Can you work these out from the model? Positions are in its coordinate system, mm. A direction names the side the tool comes from. Give positions to 0.01 mm unless a question says otherwise; leave off trailing zeros. Loops run counter-clockwise (first coordinate to the right, second up) from the corner with the lowest first, then second, coordinate; pieces in that order, holes last. Notation, with made-up numbers: (-0.75, 14.5) - (12.25, 14.5) arc R28 ccw to (12.25, 47.5) - close; hole circle Ø11 at (-21.5, 18.5). An arc over 180 degrees is marked (long way). Answer as a JSON object with one key per item and string values. Group by question number.
Item 1: Suppose I cut it at C-C on z = 7. Write out the boundary of the cut face in (x, y), and give its area (3 significant figures).
Item 2: Will these pins go through, and if not, where does the flat tip stop? pin 1 (12.5 mm diameter, centred on x = -25.5, z = -1.5, fed in from -Y); pin 2 (1.6 mm diameter, centred on x = 1, z = -3, fed in from +Y); pin 3 (1.7 mm diameter, centred on y = 3.5, z = -4.5, fed in from -X).
Item 3: Which directions (+Z, -Z, +X, -X, +Y, -Y) give clear straight access to the entire face, cutting with the end or side of a thin tool? Please do faces 4 (the flat face through (25, 3, -1.687)), 5 (the flat face through (-0.3, 2.8, -15.3)), 6 (the flat face through (-24, 4, -12.057)).
Item 4: Suppose I cut it at A-A on x = -22. Write out the boundary of the cut face in (y, z), and give its area (3 significant figures).
Item 5: Thinking about a two-plate mould opening in X: for faces 1 (the flat face through (-24, 13.04, -3)), 2 (the flat face through (-31.554, 4.42, -10.79)), 3 (the flat face through (-3, 1.6, -3)), which applies, pulls with the +X half, pulls with the -X half, needs draft (parallel to the pull), parting line crosses it, or undercut?
Item 6: Please list where these lines run through material, in increasing order: L1, parallel to X at y = 3, z = 2; L2, parallel to Y at x = -28.5, z = -2; L3, parallel to X at y = 3.5, z = -14.
Item 7: Suppose I cut it at B-B on x = 14. Write out the boundary of the cut face in (y, z).
Item 8: Suppose I cut it at D-D on y = 10. Write out the boundary of the cut face in (x, z), and give its area (3 significant figures).
from build123d import *

# Parameters (mm, degrees)
SKETCH_1_W          = 65
SKETCH_1_H          = 30.64
EXTRUDE_1_DEPTH     = 1.6
FILLET_1_R          = 2
SKETCH_2_R          = 1.35
CUT_EXTRUDE_1_DEPTH = 1.6
SKETCH_3_W          = 51.3
SKETCH_3_H          = 5
EXTRUDE_2_DEPTH     = 4
SKETCH_4_W          = 17.3
SKETCH_4_H          = 17.3
EXTRUDE_3_DEPTH     = 5.72
CHAMFER_1_SIZE      = 2.5
SKETCH_5_R          = 6.95
EXTRUDE_4_DEPTH     = 1
SKETCH_6_R          = 1.326147724
EXTRUDE_5_DEPTH     = 3.72
SKETCH_7_R          = 5.6
EXTRUDE_6_DEPTH     = 1
SKETCH_8_W          = 6.2
SKETCH_8_H          = 6.2
EXTRUDE_7_DEPTH     = 2
SKETCH_9_R          = 1.56
EXTRUDE_8_DEPTH     = 1
SKETCH_10_W         = 3.44
SKETCH_10_H         = 3
EXTRUDE_9_DEPTH     = 1.2
SKETCH_11_R         = 0.875
EXTRUDE_10_DEPTH    = 0.5


with BuildPart() as part:
    # 草图1 → 凸台-拉伸1 (new body)
    with BuildSketch(Plane(origin=(0, 0, 0), x_dir=(1, 0, 0), z_dir=(0, 1, 0))):
        with Locations((-2.796247961, 2.767463295)):
            Rectangle(SKETCH_1_W, SKETCH_1_H)
    extrude(amount=EXTRUDE_1_DEPTH)

    # 圆角1
    fillet_1_edges = [part.edges().sort_by_distance(p)[0] for p in [
        (-35.296247961, 0.8, -18.087463295),
        (29.703752039, 0.8, -18.087463295),
        (29.703752039, 0.8, 12.552536705),
        (-35.296247961, 0.8, 12.552536705),
    ]]
    fillet(fillet_1_edges, radius=FILLET_1_R)

    # 草图2 → 切除-拉伸1 (cut)
    with BuildSketch(Plane(origin=(0, 1.6, 0), x_dir=(1, 0, 0), z_dir=(0, 1, 0))):
        with Locations(Location((-32.996247961, 15.787463295, 0), (0, 0, 270))):  # turned: the seam where the file's is
            Circle(SKETCH_2_R)
        with Locations(Location((27.403752039, 15.787463295, 0), (0, 0, 270))):  # turned: the seam where the file's is
            Circle(SKETCH_2_R)
        with Locations(Location((27.403752039, -9.702536705, 0), (0, 0, 270))):  # turned: the seam where the file's is
            Circle(SKETCH_2_R)
        with Locations(Location((-32.996247961, -9.702536705, 0), (0, 0, 270))):  # turned: the seam where the file's is
            Circle(SKETCH_2_R)
    extrude(amount=-CUT_EXTRUDE_1_DEPTH, mode=Mode.SUBTRACT)

    # 草图3 → 凸台-拉伸2 (add)
    with BuildSketch(Plane.XZ):
        with Locations((-2.446247961, 8.452536705)):
            Rectangle(SKETCH_3_W, SKETCH_3_H)
    extrude(amount=EXTRUDE_2_DEPTH)

    # 草图4 → 凸台-拉伸3 (add)
    with BuildSketch(Plane(origin=(0, 1.6, 0), x_dir=(1, 0, 0), z_dir=(0, 1, 0))):
        with Locations((-24.136247961, 3.407463295)):
            Rectangle(SKETCH_4_W, SKETCH_4_H)
    extrude(amount=EXTRUDE_3_DEPTH)

    # 倒角1
    chamfer_1_edges = [part.edges().sort_by_distance(p)[0] for p in [
        (-32.786247961, 4.46, -12.057463295),
        (-32.786247961, 4.46, 5.242536705),
        (-15.486247961, 4.46, 5.242536705),
        (-15.486247961, 4.46, -12.057463295),
    ]]
    chamfer(chamfer_1_edges, length=CHAMFER_1_SIZE)

    # 草图5 → 凸台-拉伸4 (add)
    with BuildSketch(Plane(origin=(0, 7.32, 0), x_dir=(1, 0, 0), z_dir=(0, 1, 0))):
        with Locations(Location((-24.136247961, 3.407463295, 0), (0, 0, 270))):  # turned: the seam where the file's is
            Circle(SKETCH_5_R)
    extrude(amount=EXTRUDE_4_DEPTH)

    # 草图6 → 凸台-拉伸5 (add)
    with BuildSketch(Plane(origin=(0, 8.32, 0), x_dir=(1, 0, 0), z_dir=(0, 1, 0))):
        with Locations(Location((-24.136247961, 3.407463295, 0), (0, 0, 270))):  # turned: the seam where the file's is
            Circle(SKETCH_6_R)
    extrude(amount=EXTRUDE_5_DEPTH)

    # 草图7 → 凸台-拉伸6 (add)
    with BuildSketch(Plane(origin=(0, 12.04, 0), x_dir=(1, 0, 0), z_dir=(0, 1, 0))):
        with Locations(Location((-24.136247961, 3.407463295, 0), (0, 0, 270))):  # turned: the seam where the file's is
            Circle(SKETCH_7_R)
    extrude(amount=EXTRUDE_6_DEPTH)

    # 草图8 → 凸台-拉伸7 (add)
    with BuildSketch(Plane(origin=(0, 1.6, 0), x_dir=(1, 0, 0), z_dir=(0, 1, 0))):
        with Locations((-8.506247961, 3.587463295)):
            Rectangle(SKETCH_8_W, SKETCH_8_H)
        with Locations((0.963752039, 3.587463295)):
            Rectangle(SKETCH_8_W, SKETCH_8_H)
        with Locations((11.613752039, 4.787463295)):
            Rectangle(SKETCH_8_W, SKETCH_8_H)
        with Locations((18.033752039, 12.407463295)):
            Rectangle(SKETCH_8_W, SKETCH_8_H)
        with Locations((24.863752039, 4.787463295)):
            Rectangle(SKETCH_8_W, SKETCH_8_H)
        with Locations((18.033752039, -3.012536705)):
            Rectangle(SKETCH_8_W, SKETCH_8_H)
    extrude(amount=EXTRUDE_7_DEPTH)

    # 草图9 → 凸台-拉伸8 (add)
    with BuildSketch(Plane(origin=(0, 3.6, 0), x_dir=(1, 0, 0), z_dir=(0, 1, 0))):
        with Locations(Location((-8.506247961, 3.587463295, 0), (0, 0, 270))):  # turned: the seam where the file's is
            Circle(SKETCH_9_R)
        with Locations(Location((0.963752039, 3.587463295, 0), (0, 0, 270))):  # turned: the seam where the file's is
            Circle(SKETCH_9_R)
        with Locations(Location((11.613752039, 4.787463295, 0), (0, 0, 270))):  # turned: the seam where the file's is
            Circle(SKETCH_9_R)
        with Locations(Location((18.033752039, 12.407463295, 0), (0, 0, 270))):  # turned: the seam where the file's is
            Circle(SKETCH_9_R)
        with Locations(Location((24.863752039, 4.787463295, 0), (0, 0, 270))):  # turned: the seam where the file's is
            Circle(SKETCH_9_R)
        with Locations(Location((18.033752039, -3.012536705, 0), (0, 0, 270))):  # turned: the seam where the file's is
            Circle(SKETCH_9_R)
    extrude(amount=EXTRUDE_8_DEPTH)

    # 草图10 → 凸台-拉伸9 (add)
    with BuildSketch(Plane(origin=(0, 1.6, 0), x_dir=(1, 0, 0), z_dir=(0, 1, 0))):
        with Locations((-8.996247961, 14.587463295)):
            Rectangle(SKETCH_10_W, SKETCH_10_H)
        with Locations((0.443752039, 14.587463295)):
            Rectangle(SKETCH_10_W, SKETCH_10_H)
    extrude(amount=EXTRUDE_9_DEPTH)

    # 草图11 → 凸台-拉伸10 (add)
    with BuildSketch(Plane(origin=(0, 2.8, 0), x_dir=(1, 0, 0), z_dir=(0, 1, 0))):
        with Locations(Location((-8.996247961, 14.587463295, 0), (0, 0, 270))):  # turned: the seam where the file's is
            Circle(SKETCH_11_R)
        with Locations(Location((0.443752039, 14.587463295, 0), (0, 0, 270))):  # turned: the seam where the file's is
            Circle(SKETCH_11_R)
    extrude(amount=EXTRUDE_10_DEPTH)


solid = part.part
Worked out:
{
 "1": {"outline": "(-35.3, 0) - (-28.1, 0) - (-28.1, -4) - (23.2, -4) - (23.2, 0) - (29.7, 0) - (29.7, 1.6) - (-35.3, 1.6) - close", "area": "309 mm2"},
 "2": {"pin 1": "stops at y = 0", "pin 2": "stops at y = 4.6", "pin 3": "stops at x = -32.79"},
 "3": {"face 4": "+Z, +X, +Y", "face 5": "+Y", "face 6": "-Z, -X, +Y"},
 "4": {"outline": "(-4, 5.95) - (0, 5.95) - (0, -18.09) - (1.6, -18.09) - (1.6, -12.06) - (7.32, -12.06) - (7.32, -10.02) - (8.32, -10.02) - (8.32, 3.21) - (7.32, 3.21) - (7.32, 5.24) - (1.6, 5.24) - (1.6, 12.55) - (0, 12.55) - (0, 10.95) - (-4, 10.95) - close; (12.04, -8.58) - (13.04, -8.58) - (13.04, 1.77) - (12.04, 1.77) - close", "area": "192 mm2"},
 "5": {"face 1": "needs draft", "face 2": "pulls with the -X half", "face 3": "undercut"},
 "6": {"L1": "x = -32.79 to -15.49, 14.93 to 21.13", "L2": "y = 0 to 8.32, 12.04 to 13.04", "L3": "x = 14.93 to 21.13"},
 "7": {"outline": "(-4, 5.95) - (0, 5.95) - (0, -18.09) - (1.6, -18.09) - (1.6, -7.89) - (3.6, -7.89) - (3.6, -1.69) - (1.6, -1.69) - (1.6, 12.55) - (0, 12.55) - (0, 10.95) - (-4, 10.95) - close"},
 "8": {"outline": "circle Ø2.65 at (-24.14, -3.41)", "area": "5.53 mm2"}
}
